Verification items for the finished model (mm, model axes). A direction names the side the tool comes from. Give positions to 0.01 mm unless a question says otherwise; leave off trailing zeros. Order: outer loops, then holes, each group sorted by start corner. A loop starts at its lowest first (then second) coordinate and runs counter-clockwise, first axis right, second up.
from build123d import *

# Parameters (mm, degrees)
F0_W     = 65
F0_H     = 40
F1_DEPTH = 3
F3_DEPTH = 40
F4_W     = 3.5
F4_H     = 2
F5_DEPTH = 40
F6_W     = 10.0229219794
F6_H     = 7.5
F6_W_2   = 13.6237391531
F7_DEPTH = 65
F8_R     = 5
F9_R     = 5
F10_R    = 2
F11_R    = 10


with BuildPart() as f1:
    # F0 (on Front) → F1 (new body)
    with BuildSketch(Plane.XZ):
        Rectangle(F0_W, F0_H)
    extrude(amount=F1_DEPTH)

    # F2 (on face) → F3 (join, through all)
    with BuildSketch(Plane.XY.offset(20)):
        with BuildLine():
            ThreePointArc((32.5, 2.100319489), (16.2838980434, 0.5256269687), (0, 0))
            Line((0, 0), (32.5, 0))
            Line((32.5, 0), (32.5, 2.100319489))
        make_face()
        with BuildLine():
            ThreePointArc((0, 0), (-16.2838980434, 0.5256269687), (-32.5, 2.100319489))
            Line((-32.5, 2.100319489), (-32.5, 0))
            Line((-32.5, 0), (0, 0))
        make_face()
    extrude(amount=-F3_DEPTH)

    # F4 (on face) → F5 (join, through all)
    with BuildSketch(Plane(origin=(0, 0, -20), x_dir=(1, 0, 0), z_dir=(0, 0, -1))):
        Polygon((-17, 10.6432288885), (-17, 3), (-14, 3), (-14, 7.6432288885), (-11.5, 7.6432288885), (-11.5, 10.6432288885), align=None)
        Polygon((14, 3), (17, 3), (17, 10.7397525311), (11.5, 10.7397525311), (11.5, 7.7397525311), (14, 7.7397525311), align=None)
        with Locations((0, 4)):
            Rectangle(F4_W, F4_H)
    extrude(amount=-F5_DEPTH)

    # F6 (on face) → F7 (cut, through all)
    with BuildSketch(Plane.YZ.offset(32.5)):
        with Locations((-8.0114609897, -16.25)):
            Rectangle(F6_W, F6_H)
        with Locations((-9.8118695766, 16.25)):
            Rectangle(F6_W_2, F6_H)
    extrude(amount=-F7_DEPTH, mode=Mode.SUBTRACT)

    # F8
    f8_edges = [f1.edges().sort_by_distance(p)[0] for p in [
        (17, -3, 0),
        (-17, -3, 0),
    ]]
    fillet(f8_edges, radius=F8_R)

    # F9
    f9_edges = [f1.edges().sort_by_distance(p)[0] for p in [
        (11.5, -9.239753, 12.5),
        (-11.5, -9.143229, 12.5),
        (11.5, -9.239753, -12.5),
        (-11.5, -9.143229, -12.5),
    ]]
    fillet(f9_edges, radius=F9_R)

    # F10
    f10_edges = [f1.edges().sort_by_distance(p)[0] for p in [
        (17, -10.739753, 0),
        (-17, -10.643229, 0),
    ]]
    fillet(f10_edges, radius=F10_R)

    # F11
    f11_edges = [f1.edges().sort_by_distance(p)[0] for p in [
        (32.5, -0.44984, 20),
        (-32.5, -0.44984, 20),
    ]]
    fillet(f11_edges, radius=F11_R)


solid = f1.part
(1) Release check for a two-part mould opening along X. For faces 6 (the flat face through (-32.5, 0, -5)), 7 (the flat face through (0, -4, 12.5)), 8 (the cylindrical face through (-14.34, -7.62, -12.01)), 9 (the flat face through (-14, -5, 0)) record: pulls with the +X half, pulls with the -X half, needs draft (parallel to the pull), parting line crosses it, or undercut.
Solved:
face 6: pulls with the -X half
face 7: needs draft
face 8: undercut
face 9: undercut
(2) Section check A-A, the plane y = -6.5. Enter the section's corners in (x, z), then the cut area to 3 significant figures.
Solved:
outline: (-17.23, -12.5) - (-16.5, -12.5) arc R5 ccw to (-14, -11.83) - (-14, 11.83) arc R5 ccw to (-16.5, 12.5) - (-17.23, 12.5) - close; (14, -11.83) arc R5 ccw to (16.5, -12.5) - (17.23, -12.5) - (17.23, 12.5) - (16.5, 12.5) arc R5 ccw to (14, 11.83) - close
area: 159 mm2
(3) Set-up check for faces 1 (the cylindrical face through (13.587, -8.644, -11.564)), 2 (the flat face through (1.75, -4, 0)), 3 (the cylindrical face through (13.587, -8.644, 11.564)), 4 (the flat face through (0, -4, -12.5)), 5 (the flat face through (-13, -7.643, 0)): record each of +Z, -Z, +X, -X, +Y, -Y from which the full face is reachable in a straight line by a thin tool's end or side.
Solved:
face 1: -Z, -Y
face 2: +Z, -Z, -Y
face 3: +Z, -Y
face 4: -Z, +X, -X, -Y
face 5: +Z, -Z
(4) Scan lines: line 1 (X direction, y = -4.5, z = -5); line 2 (Z direction, x = -0.5, y = -3.5); line 3 (X direction, y = -3.5, z = -10). Record each from-to range of solid material in increasing order.
Solved:
line 1: x = -18.43 to -14, -1.75 to 1.75, 14 to 18.43
line 2: z = -12.5 to 12.5
line 3: x = -19.82 to -14, -1.75 to 1.75, 14 to 19.82
(5) Go/stop test with flat-tipped pins: pin 1 (1 mm diameter, centred on x = 1, z = 0.5, fed in from -Y); pin 2 (1 mm diameter, centred on x = -13, z = -6, fed in from -Y); pin 3 (1.6 mm diameter, centred on x = 0.5, y = -4.5, fed in from +Z); pin 4 (4.5 mm diameter, centred on x = 20, y = -7.5, fed in from +Z). Record where each tip stops, or that it passes through.
Solved:
pin 1: stops at y = -5
pin 2: stops at y = -10.64
pin 3: stops at z = 12.5
pin 4: passes through
(6) Section check C-C, the plane x = -19.5. Enter the section's corners in (y, z).
Solved:
outline: (-3.67, -12.5) - (-3, -12.5) - (-3, -20) - (0.75, -20) - (0.75, 20) - (-3, 20) - (-3, 12.5) - (-3.67, 12.5) - close
(7) Section check B-B, the plane z = 6. Enter the section's corners in (x, y), then the cut area to 3 significant figures.
Solved:
outline: (-32.5, -3) - (-22, -3) arc R5 cw to (-17, -8) - (-17, -8.64) arc R2 ccw to (-15, -10.64) - (-11.5, -10.64) - (-11.5, -7.64) - (-14, -7.64) - (-14, -3) - (-1.75, -3) - (-1.75, -5) - (1.75, -5) - (1.75, -3) - (14, -3) - (14, -7.74) - (11.5, -7.74) - (11.5, -10.74) - (15, -10.74) arc R2 ccw to (17, -8.74) - (17, -8) arc R5 cw to (22, -3) - (32.5, -3) - (32.5, 2.1) arc R252.5 cw to (-32.5, 2.1) - close
area: 318 mm2
(8) Section check D-D, the plane y = -1.75. Enter the section's corners in (x, z).
Solved:
outline: (-32.5, -20) - (32.5, -20) - (32.5, 10) arc R10 ccw to (22.5, 20) - (-22.5, 20) arc R10 ccw to (-32.5, 10) - close
